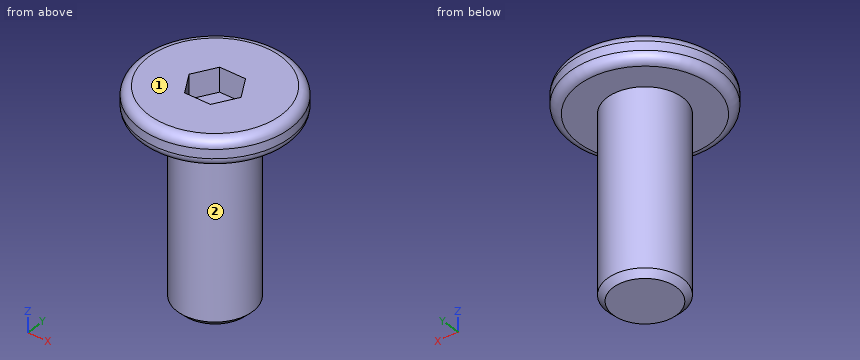
```python
from build123d import *

# Parameters (mm, degrees)
SKETCH_1_R          = 2.5
EXTRUDE_1_DEPTH     = 0.45
SKETCH_2_R          = 1.25
EXTRUDE_2_DEPTH     = 6
CHAMFER_1_SIZE      = 0.2
CUT_EXTRUDE_1_DEPTH = 0.8
FILLET_2_R          = 0.3


with BuildPart() as part:
    # 草图1 → 凸台-拉伸1 (new body, symmetric)
    with BuildSketch(Plane.XY):
        Circle(SKETCH_1_R)
    extrude(amount=EXTRUDE_1_DEPTH, both=True)

    # 草图2 → 凸台-拉伸2 (add)
    with BuildSketch(Plane(origin=(0, 0, -0.45), x_dir=(-1, 0, 0), z_dir=(0, 0, -1))):
        Circle(SKETCH_2_R)
    extrude(amount=EXTRUDE_2_DEPTH)

    # 倒角1
    chamfer_1_edges = [part.edges().sort_by_distance(p)[0] for p in [
        (1.25, 0, -6.45),
    ]]
    chamfer(chamfer_1_edges, length=CHAMFER_1_SIZE)

    # 草图3 → 切除-拉伸1 (cut)
    with BuildSketch(Plane.XY.offset(0.45)):
        Polygon((0.866025404, 0), (0.433012702, 0.75), (-0.433012702, 0.75), (-0.866025404, 0), (-0.433012702, -0.75), (0.433012702, -0.75), align=None)
    extrude(amount=-CUT_EXTRUDE_1_DEPTH, mode=Mode.SUBTRACT)

    # 圆角2
    fillet_2_edges = [part.edges().sort_by_distance(p)[0] for p in [
        (-2.5, 0, -0.45),
        (-2.5, 0, 0.45),
    ]]
    fillet(fillet_2_edges, radius=FILLET_2_R)


solid = part.part
```
Work out the finished part from the listing and answer in its coordinate system (mm). Face numbers are marked on the shaded views. A direction names the side the tool comes from. Give positions to 0.01 mm unless a question says otherwise; leave off trailing zeros. Loops run counter-clockwise (first coordinate to the right, second up) from the corner with the lowest first, then second, coordinate; pieces in that order, holes last. Notation, with made-up numbers: (31.25, 17) - (61.25, 17) arc R29 cw to (61.25, 37) - close; hole circle Ø3 at (-12, 25). An arc over 180 degrees is marked (long way). One line per question, with ' | ' between items.
(1) Straight lines are drawn through the part: probe 1 along Z at (x, y) = (-1.85, 0.1); probe 2 along X at (y, z) = (1, -5.5); probe 3 along Z at (x, y) = (-0.35, -0.15). For each, find the intervals that lie inside material, in ascending order.
Recorded:
probe 1: z = -0.45 to 0.45 | probe 2: x = -0.75 to 0.75 | probe 3: z = -6.45 to -0.35
(2) The part is cut by section C-C (z = -2.5). Write down the section's boundary in (x, y), then the cut area to 3 significant figures.
Recorded:
outline: circle Ø2.5 at (0, 0) | area: 4.91 mm²
(3) The part is cut by section A-A (x = 0). Write down the section's boundary in (y, z), then the cut area to 3 significant figures.
Recorded:
outline: (-2.5, -0.15) arc R0.3 ccw to (-2.2, -0.45) - (-1.25, -0.45) - (-1.25, -6.25) - (-1.05, -6.45) - (1.05, -6.45) - (1.25, -6.25) - (1.25, -0.45) - (2.2, -0.45) arc R0.3 ccw to (2.5, -0.15) - (2.5, 0.15) arc R0.3 ccw to (2.2, 0.45) - (0.75, 0.45) - (0.75, -0.35) - (-0.75, -0.35) - (-0.75, 0.45) - (-2.2, 0.45) arc R0.3 ccw to (-2.5, 0.15) - close | area: 18.2 mm²
(4) Each of these flat-tipped pins is pushed along its axis until it touches: pin 1 Ø1 at (y, z) = (-1, -3) entering from +X; pin 2 Ø3 at (x, y) = (-2, -2) entering from -Z; pin 3 Ø1 at (y, z) = (-1.5, -3) entering from +X. Where does it stop, or does it pass through?
Recorded:
pin 1: stops at x = 1.15 | pin 2: stops at z = -0.45 | pin 3: stops at x = 0.75
(5) The part is cut by section B-B (z = 0.25). Write down the section's boundary in (x, y), then the cut area to 3 significant figures.
Recorded:
outline: circle Ø4.97 at (0, 0); hole (-0.87, 0) - (-0.43, -0.75) - (0.43, -0.75) - (0.87, 0) - (0.43, 0.75) - (-0.43, 0.75) - close | area: 17.4 mm²
(6) A tool of negligible diameter and unlimited length cuts with its end or side. For the marked faces 1 and 2, from which of +Z, -Z, +X, -X, +Y, -Y can it reach the whole face along a straight path? Write none if from no direction.
Recorded:
face 1: +Z, +X, -X, +Y, -Y | face 2: -Z
